Geometry: see drawing. Coordinates: mm, zero at the bounding-box minimum. A direction names the side the tool comes from. Give positions to 0.01 mm unless a question says otherwise; leave off trailing zeros. Loops run counter-clockwise (first coordinate to the right, second up) from the corner with the lowest first, then second, coordinate; pieces in that order, holes last. Notation, with made-up numbers: (42.5, -31.5) -> (90.5, -31.5) arc R15 cw to (90.5, -9.5) -> close; hole circle Ø7 at (62, -29.5). An arc over 180 degrees is marked (long way). Return JSON: item names as keys, results as strings. Group by question number.
(1) Cut plane A-A on y = 21.5. Return loops of the section in (x, z), then the cut area to 3 significant figures.
(2) Cut plane B-B on x = 5.5. Return loops of the section in (y, z).
(3) Ray query, line 1 (Y direction, x = 12, z = 18.9); line 2 (Z direction, x = 3, y = 20.5); line 3 (Y direction, x = 12, z = 3). Return the intervals inside material, ascending. Write a range as from..to.
(4) Draft query along Y for the marked faces 1, 2 and 3. Return one class per face: released by +Y, released by -Y, zero draft, split by the parting line, or undercut.
(5) Pin query (flat end, axial travel): pin 1 (2 mm diameter, centred on y = 19.5, z = 2, fed in from +X); pin 2 (8 mm diameter, centred on x = 12, y = 21.5, fed in from -Z); pin 3 (6 mm diameter, centred on x = 21, z = 9, fed in from +Y); pin 4 (5.5 mm diameter, centred on y = 3.5, z = 14.5, fed in from -X). Return the tip coordinate at first contact, or that it passes through.
(6) Cut plane D-D on z = 10. Return loops of the section in (x, y), then the cut area to 3 significant figures.
(7) Cut plane C-C on x = 15.5. Return loops of the section in (y, z), then the cut area to 3 significant figures.
(8) Access query for the marked faces 4, 5, 6 and 7. Directions: +Z, -Z, +X, -X, +Y, -Y. A direction counts if a zero-diameter tool reaches every point of the face in a straight line with its end or side. Return the directions, or none.
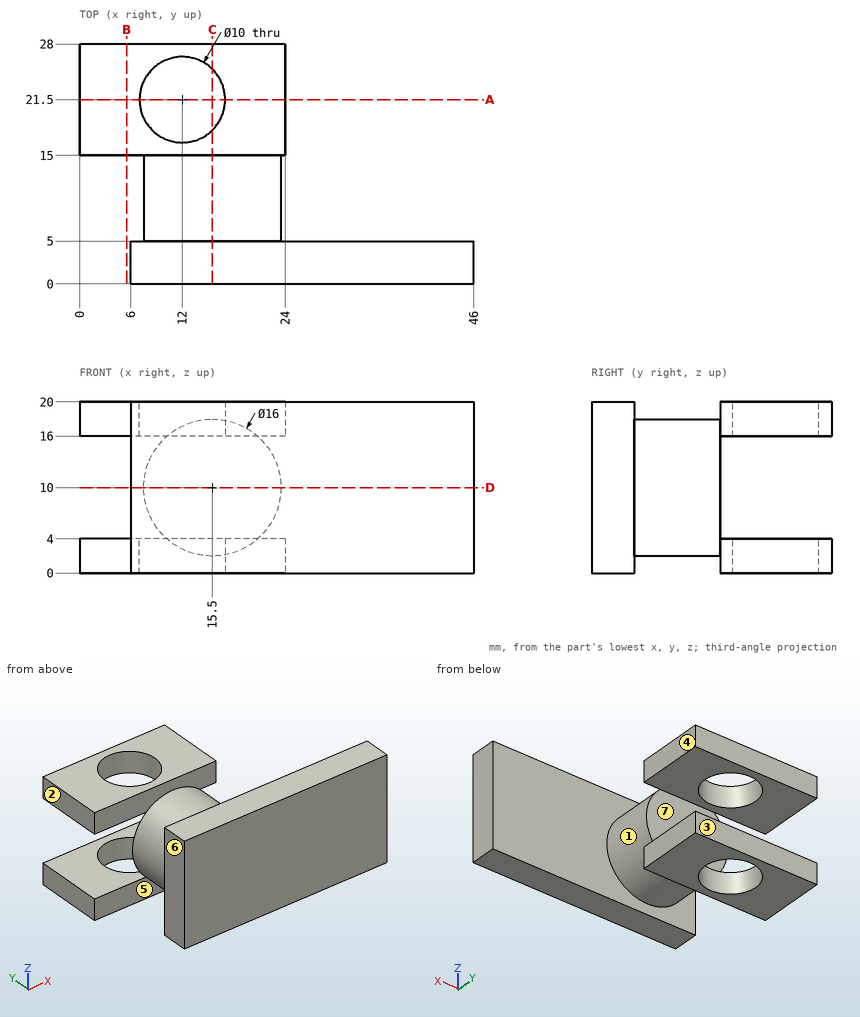
Answers:
{
 "1": {"outline": "(0, 0) -> (7, 0) -> (7, 4) -> (0, 4) -> close; (0, 16) -> (7, 16) -> (7, 20) -> (0, 20) -> close; (17, 0) -> (24, 0) -> (24, 4) -> (17, 4) -> close; (17, 16) -> (24, 16) -> (24, 20) -> (17, 20) -> close", "area": "112 mm²"},
 "2": {"outline": "(15, 0) -> (28, 0) -> (28, 4) -> (15, 4) -> close; (15, 16) -> (28, 16) -> (28, 20) -> (15, 20) -> close"},
 "3": {"line 1": "0..5, 15..16.5, 26.5..28", "line 2": "0..4, 16..20", "line 3": "0..16.5, 26.5..28"},
 "4": {"face 1": "undercut", "face 2": "zero draft", "face 3": "released by +Y"},
 "5": {"pin 1": "x = 24", "pin 2": "through", "pin 3": "y = 15", "pin 4": "x = 6"},
 "6": {"outline": "(6, 0) -> (46, 0) -> (46, 5) -> (23.5, 5) -> (23.5, 15) -> (7.5, 15) -> (7.5, 5) -> (6, 5) -> close", "area": "360 mm²"},
 "7": {"outline": "(0, 0) -> (5, 0) -> (5, 2) -> (15, 2) -> (15, 0) -> (17.93, 0) -> (17.93, 4) -> (15, 4) -> (15, 16) -> (17.93, 16) -> (17.93, 20) -> (15, 20) -> (15, 18) -> (5, 18) -> (5, 20) -> (0, 20) -> close; (25.07, 0) -> (28, 0) -> (28, 4) -> (25.07, 4) -> close; (25.07, 16) -> (28, 16) -> (28, 20) -> (25.07, 20) -> close", "area": "307 mm²"},
 "8": {"face 4": "+Z, -Z, +X, +Y", "face 5": "-Z", "face 6": "+Z, -Z, -X, -Y", "face 7": "+X, -X, +Y"}
}
